Build history of the part. All positions in model axes, mm. Face numbers are marked on the shaded views. Give positions to 0.01 mm unless a question says otherwise; leave off trailing zeros. Order: outer loops, then holes, each group sorted by start corner. A loop starts at its lowest first (then second) coordinate and runs counter-clockwise, first axis right, second up. Notation, with made-up numbers: M 43,22.5 L 79,22.5 A26 cw 79,52.5 Z; hole C 26.25,-14.75 d7. An arc over 180 degrees is marked long. Use CSV: the item, a comma, the result in double quotes. Start each with the question number.
Item 1: Band-saw the part on A-A on y = 4.25. Write the cut outline in (x, z), plus the area to 3 significant figures.
Item 2: Two-plate mould, pull along Z, no slides. Class the marked faces 1, 2, 3 and 4: pulls with the +Z half, pulls with the -Z half, needs draft (parallel to the pull), parting line crosses it, or undercut.
Item 3: Wall check: line 1 along Y through (x, z) = (-0.4, 0.25); line 2 along Z through (x, y) = (0, 2.75); line 3 along Y through (x, z) = (1.05, 1.25). Give the ranges that are in metal, low to high.
Item 4: Band-saw the part on C-C on y = 25.25. Write the cut outline in (x, z).
Item 5: Pin check, flat tips, straight feed: P1, Ø2, axis at y = 20, z = 1, coming from the +X side; P2, Ø2, axis at x = -2, z = -1, coming from the +Y side; P3, Ø1.5, axis at x = -0.5, z = 0, coming from the -Y side. Stop position of each tip, or through.
Item 6: Band-saw the part on B-B on y = 12.25. Write the cut outline in (x, z).
from build123d import *

# Parameters (mm, degrees)
BOSS_EXTRUDE1_DEPTH = 20
SKETCH2_R           = 1.5
BOSS_EXTRUDE2_DEPTH = 7
SKETCH3_R           = 1.5
CUT_EXTRUDE1_DEPTH  = 7
FILLET1_R           = 1


with BuildPart() as part:
    # Sketch1 → Boss-Extrude1 (new body)
    with BuildSketch(Plane(origin=(0, 0, 0), x_dir=(1, 0, 0), z_dir=(0, 1, 0))):
        Polygon((2.214824591, -1.851454932), (2.7108193, 0.992366895), (0.495994709, 2.843821827), (-2.214824591, 1.851454932), (-2.7108193, -0.992366895), (-0.495994709, -2.843821827), align=None)
    extrude(amount=BOSS_EXTRUDE1_DEPTH)

    # Sketch2 → Boss-Extrude2 (add)
    with BuildSketch(Plane(origin=(0, 20, 0), x_dir=(1, 0, 0), z_dir=(0, 1, 0))):
        Circle(SKETCH2_R)
    extrude(amount=BOSS_EXTRUDE2_DEPTH)

    # Sketch3 → Cut-Extrude1 (cut)
    with BuildSketch(Plane.XZ):
        Circle(SKETCH3_R)
    extrude(amount=-CUT_EXTRUDE1_DEPTH, mode=Mode.SUBTRACT)

    # Fillet1
    fillet1_edges = [part.edges().sort_by_distance(p)[0] for p in [
        (-1.5, 27, 0),
    ]]
    fillet(fillet1_edges, radius=FILLET1_R)


solid = part.part
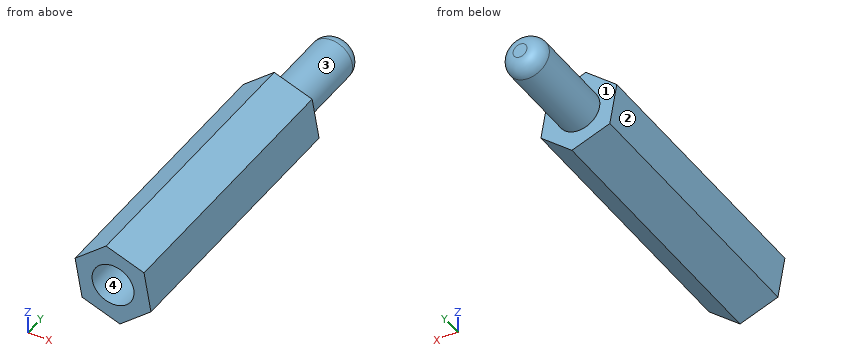
Model answer:
1,outline,"M -2.71,0.99 L -2.21,-1.85 L 0.5,-2.84 L 2.71,-0.99 L 2.21,1.85 L -0.5,2.84 Z; hole C 0,0 d3"
1,area,"14.6 mm^2"
2,face 1,"needs draft"
2,face 2,"pulls with the -Z half"
2,face 3,"parting line crosses it"
2,face 4,"undercut"
3,line 1,"y = 7 to 27"
3,line 2,"z = -2.66 to -1.5, 1.5 to 2.66"
3,line 3,"y = 0 to 20"
4,outline,"C 0,0 d3"
5,P1,"stops at x = 2.54"
5,P2,"stops at y = 26.68"
5,P3,"stops at y = 7"
6,outline,"M -2.71,0.99 L -2.21,-1.85 L 0.5,-2.84 L 2.71,-0.99 L 2.21,1.85 L -0.5,2.84 Z"
